The figure shows three views and two pictorial views of one solid part (mm, origin at its lowest corner). Answer the questions. A direction names the side the tool comes from. Coordinates: 2 decimals unless noted, no trailing zeros. Write each loop counter-clockwise with the first axis right and the second up, starting at its lowest first coordinate (ties: lowest second). Pieces come first, ordered by that corner, then holes. Notation, with made-up numbers: M -11,-11.75 L 7,-11.75 A32 ccw 7,14.25 Z; hole C -18,-8 d11. An arc over 180 degrees is marked long. Write item = value, one per line.
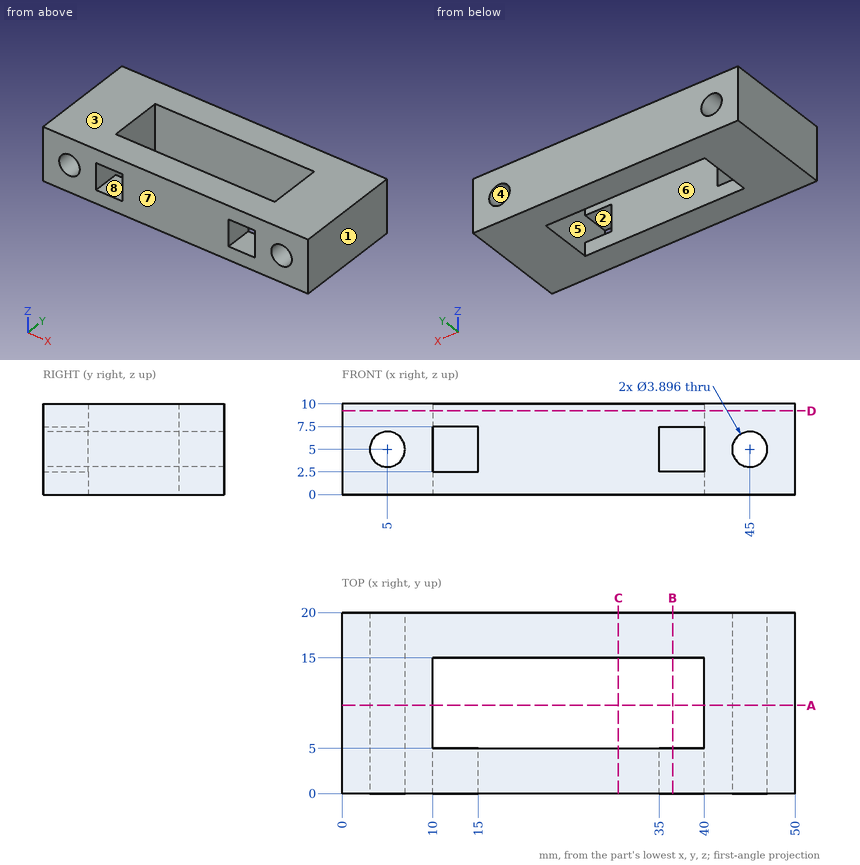
Item 1: Which of the six approach directions +Z, -Z, +X, -X, +Y, -Y give full straight-line access (tool end or side, diameter ignored) to the marked faces 4, 5, 6, 7 and 8?
Worked answers:
face_4 = +Y, -Y
face_5 = none
face_6 = +Z, -Z
face_7 = +Z, -Z, +X, -X, -Y
face_8 = -Y
Item 2: Find section C-C (x = 30.5). Determine the outline of the cut face in (y, z), and give its area (3 significant figures).
Worked answers:
outline = M 0,0 L 5,0 L 5,10 L 0,10 Z; M 15,0 L 20,0 L 20,10 L 15,10 Z
area = 100 mm²
Item 3: Find section D-D (z = 9.25). Determine the outline of the cut face in (x, y).
Worked answers:
outline = M 0,0 L 50,0 L 50,20 L 0,20 Z; hole M 10,5 L 40,5 L 40,15 L 10,15 Z
Item 4: Find section A-A (y = 9.75). Determine the outline of the cut face in (x, z), and give its area (3 significant figures).
Worked answers:
outline = M 0,0 L 10,0 L 10,10 L 0,10 Z; M 40,0 L 50,0 L 50,10 L 40,10 Z; hole C 5,5 d3.9; hole C 45,5 d3.9
area = 176 mm²
Item 5: Consider line 1 along Y through (x, z) = (33, 0.75); line 2 along Z through (x, y) = (45, 11); line 3 along X through (y, z) = (11, 9). Determine where each line is inside the solid, lowest interval first. Write a range as from..to.
Worked answers:
line_1 = 0..5, 15..20
line_2 = 0..3.05, 6.95..10
line_3 = 0..10, 40..50
Item 6: Find section B-B (x = 36.5). Determine the outline of the cut face in (y, z), and give its area (3 significant figures).
Worked answers:
outline = M 0,0 L 5,0 L 5,2.5 L 0,2.5 Z; M 0,7.5 L 5,7.5 L 5,10 L 0,10 Z; M 15,0 L 20,0 L 20,10 L 15,10 Z
area = 75.0 mm²
Item 7: For a pull along X with two mould halves and no side action, classify the marked faces 1, 2 and 3 as released by +X, released by -X, zero draft, split by the parting line, or undercut.
Worked answers:
face_1 = released by +X
face_2 = undercut
face_3 = zero draft
